Can you work these out from the model? Positions are in its coordinate system, mm. Round coordinates to 2 decimals unless told otherwise and drop trailing zeros. Write each loop counter-clockwise with the first axis right and the second up, starting at its lowest first coordinate (ties: lowest second). Pieces come first, ordered by that corner, then holes.
Q1. Please list where these lines run through material, in increasing order: line 1 along X through (y, z) = (-46, -0.55); line 2 along X through (y, z) = (-134.5, -1.25); line 3 along Y through (x, z) = (109.5, -1.8).
Q2. If we section it at C-C (y = -87.5): Please give me the cut outline in (x, z), plus the area to 3 significant figures.
Q3. If we section it at A-A (z = -2.55): Give the number of separate pieces and of enclosed holes in the cut face, plus the area to 3 significant figures.
Q4. If we section it at B-B (x = 0): Please give me the cut outline in (y, z), plus the area to 3 significant figures.
Q5. I'm going to push flat-ended pins straight in: pin 1 Ø13 at (x, y) = (-47.294, 48.706) entering from +Z; pin 2 Ø0.9 at (y, z) = (132.5, -1) entering from -X; pin 3 Ø1.5 at (y, z) = (54.5, -1) entering from +X; pin 4 Ø1.5 at (y, z) = (-172.5, -1.5) entering from +X. Where does each tip first touch, or does it pass through?
Autodesk Fusion 360 part; units mm, degrees
sketch "Sketch1" plane through (0, 0, 0) normal (0, 0, -1) x (1, 0, 0)
  circle A0 centre (0, 0) radius 240
  line L0 (0.0048, -240) -> (125.0048, -240)
  line L1 (125.0048, -240) -> (125.0048, -204.8751)
  line L2 (1.5986, 239.9947) -> (1.5986, -147.0053)
  line L3 (125.0048, -204.8751) -> (-125.0048, -204.8751)
  arc A1 (125.0048, -204.8751) -> (-125.0048, -204.8751) centre (0, -310.93) ccw
  circle A2 centre (-47.294, 47.294) radius 5
  line L4 (-47.294, 47.294) -> (48.706, 47.294)
  line L5 (48.706, 47.294) -> (48.706, -48.706)
  line L6 (48.706, -48.706) -> (-47.294, -48.706)
  line L7 (-47.294, -48.706) -> (-47.294, 47.294)
  circle A3 centre (48.706, 47.294) radius 5
  circle A4 centre (48.706, -48.706) radius 5
  circle A5 centre (-47.294, -48.706) radius 5
  line L8 (1.5986, 239.9947) -> (251.5986, 239.9947)
  line L9 (-47.294, 47.294) -> (-47.294, 235.294)
  line L10 (-47.294, 47.294) -> (-235.294, 47.294)
  line L11 (105.5391, 215.5493) -> (105.5391, 169.5493)
  line L12 (105.5391, 169.5493) -> (105.5391, 109.5493)
  line L13 (105.5391, 109.5493) -> (213.5391, 109.5493)
  line L14 (105.5391, 109.5493) -> (105.5391, 124.5493)
  line L15 (105.5391, 169.5493) -> (105.5391, 154.5493)
  line L16 (120.5391, 124.5493) -> (120.5391, 154.5493)
  arc A6 (120.5391, 154.5493) -> (90.5391, 154.5493) centre (105.5391, 154.5493) ccw
  line L17 (90.5391, 154.5493) -> (90.5391, 124.5493)
  arc A7 (90.5391, 124.5493) -> (120.5391, 124.5493) centre (105.5391, 124.5493) ccw
  line L18 (105.5391, 124.5493) -> (105.5391, 154.5493) construction
  line L19 (1.5986, -147.0053) -> (41.5986, -147.0053)
  line L20 (41.5986, -147.0053) -> (41.5986, -152.3633)
  line L21 (1.5986, -147.0053) -> (1.5986, -115.0053)
  line L22 (1.5986, -115.0053) -> (-38.4014, -115.0053)
  line L23 (41.5986, -152.3633) -> (-38.4014, -152.3633)
  line L24 (-38.4014, -152.3633) -> (-38.4014, -115.0053)
  line L25 (-38.4014, -115.0053) -> (41.5986, -115.0053)
  line L26 (41.5986, -115.0053) -> (41.5986, -152.3633)
  line L27 (-145.8667, 190.5857) -> (-145.8667, 148.0857)
  line L28 (-145.8667, 148.0857) -> (-188.8667, 148.0857)
  circle A8 centre (-145.8667, 148.0857) radius 5
  line L29 (-145.8667, 148.0857) -> (-110.8667, 148.0857)
  line L30 (-110.8667, 159.0843) -> (-110.8667, 124.0843)
  line L31 (-125.8667, 159.0843) -> (-125.8667, 124.0843)
  arc A9 (-125.8667, 124.0843) -> (-95.8667, 124.0843) centre (-110.8667, 124.0843) ccw
  line L32 (-95.8667, 124.0843) -> (-95.8667, 159.0843)
  arc A10 (-95.8667, 159.0843) -> (-125.8667, 159.0843) centre (-110.8667, 159.0843) ccw
  line L33 (-110.8667, 159.0843) -> (-110.8667, 124.0843) construction
  line L34 (-110.8667, 148.0857) -> (-110.8667, 159.0843)
  line L35 (-107.1508, -115.0053) -> (-107.5583, -130.5)
  circle A11 centre (-107.5583, -130.5) radius 5
  line L36 (-38.4014, -115.0053) -> (-210.6508, -115.0053)
  line L37 (-210.6508, -115.0053) -> (-107.1508, -115.0053)
  line L38 (152.5158, 185.3077) -> (67.5158, 185.3077)
  line L39 (67.5158, 185.3077) -> (67.5158, 230.3077)
  line L40 (-107.5583, -130.5) -> (107.9417, -130.5)
  circle A12 centre (107.9417, -130.5) radius 5
  line L41 (-145.8667, 148.0857) -> (149.1333, 148.0857)
  circle A13 centre (149.1333, 148.0857) radius 5
  dimension "d1" = 480
  dimension "d2" = 125
  dimension "d3" = 387
  dimension "d7" = 10
  dimension "d8" = 96
  dimension "d9" = 96
  dimension "d10" = 10
  dimension "d11" = 10
  dimension "d12" = 10
  dimension "d13" = 250
  dimension "d14" = 188
  dimension "d15" = 188
  dimension "d16" = 46
  dimension "d17" = 60
  dimension "d18" = 108
  dimension "d19" = 15
  dimension "d20" = 15
  dimension "d21" = 30
  dimension "d22" = 40
  dimension "d23" = 32
  dimension "d24" = 40
  dimension "d25" = 42.5
  dimension "d26" = 43
  dimension "d27" = 10
  dimension "d28" = 35
  dimension "d29" = 35
  dimension "d30" = 30
  dimension "d32" = 15.5
  dimension "d33" = 10
  dimension "d34" = 103.5
  dimension "d35" = 85
  dimension "d36" = 45
  dimension "d40" = 215.5
  dimension "d41" = 10
  dimension "d42" = 295
  dimension "d43" = 10
extrude "Extrude3" add sketch "Sketch1" along normal blind 3 contours A0 L2 A1 L4 L5 L6 A3 A4 L13 L17 A7 L20 L25 L26 L41 | A0 L11 L13 L16 A6 A7 L38 | A0 L11 L38 | A0 A1 L24 L35 A11 L36 L37 L40 | A0 L11 L38 L39 | A0 L2 L11 A6 L17 L38 L39 L41 | A0 L2 A2 L6 L7 A5 L10 L22 L25 L36 L37 | A0 A2 L9 L10 L28 A8 L29 L31 A9 L32 L41 | L24 L35 A11 L36 L40 | A0 L2 L9 L41 | L2 A2 L4 L9 L41 | A0 L27 L28 A8 | A0 L9 L27 A8 L29 L31 L32 A10 L41 | L2 L4 L5 L6 A3 A4 | L2 A2 L4 L6 L7 A5
equation "d2 = ( 250 / 2 ) * 1 mm"
equation "d3 = 355 mm + 32 mm"
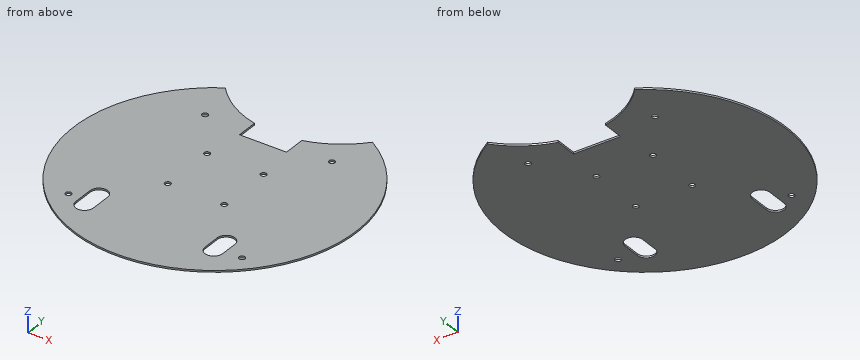
A:
1. line 1: x = -235.55 to -52.12, -42.46 to 43.88, 53.54 to 235.55
1. line 2: x = -198.77 to -125.87, -95.87 to 90.54, 120.54 to 198.77
1. line 3: y = -213.56 to -169.02, -110.08 to 125.75, 135.25 to 188.93
2. outline: (-223.48, -3) - (223.48, -3) - (223.48, 0) - (-223.48, 0) - close
2. area: 1,340 mm2
3. separate pieces: 1
3. enclosed holes: 10
3. area: 158,000 mm2
4. outline: (-240, -3) - (115.01, -3) - (115.01, 0) - (-240, 0) - close
4. area: 1,070 mm2
5. pin 1: stops at z = 0
5. pin 2: stops at x = -200.41
5. pin 3: stops at x = 233.9
5. pin 4: stops at x = 167.64
